Could you check a few things on this model? Use its own coordinates, in mm. A direction names the side the tool comes from. Give positions to 0.01 mm unless a question says otherwise; leave off trailing zeros. Order: outer loops, then holes, each group sorted by start corner. A loop starts at its lowest first (then second) coordinate and runs counter-clockwise, first axis right, second up. Notation, with made-up numbers: (44.25, 60) - (71.25, 60) arc R32 cw to (71.25, 91) - close; hole circle Ø4 at (39, 27). An arc over 180 degrees is marked (long way). One line per question, with ' | ' between items. Start each with the question number.
1. Imagine slicing it at B-B (x = 9). Please give me the cut outline in (y, z), and give its area (3 significant figures).
2. Which directions (+Z, -Z, +X, -X, +Y, -Y) give clear straight access to the entire face, cutting with the end or side of a thin tool? Please do faces 5 (the flat face through (50, -1, 12)), 6 (the flat face through (-1, -40, 24)).
3. For P1, Ø4, axis at x = 21.5, y = -9.5, coming from the +Z side; P2, Ø10, axis at x = -36.5, y = -38.5, coming from the -Z side, each with a flat end and sliding along its axis, tell me the tip position at first contact or that it passes through.
4. I need wall thicknesses on probe 1 along X at (y, z) = (18, 4); probe 2 along Z at (x, y) = (-21, 46.5). Which ranges of each line are inside material? Lowest first, please. Write a range as from..to.
5. Imagine slicing it at D-D (z = 20.25). Please give me the cut outline in (x, y).
6. Imagine slicing it at C-C (y = -26). Please give me the cut outline in (x, z), and give its area (4 significant figures).
7. If we mould it in two halves opening along Z, with no side actions, what happens to faces 1 (the flat face through (-1, 50, 12)), 2 (the flat face through (0, 49, 25)), 3 (the flat face through (-1, -47.5, 9)), 4 (the cylindrical face through (0.665, -45.361, 20.245))? For each: released by +Z, released by -Z, zero draft, split by the parting line, or undercut.
8. Imagine slicing it at A-A (z = 8). Please give me the cut outline in (x, y).
```python
from build123d import *

# Parameters (mm, degrees)
F0_W     = 100
F0_H     = 100
F1_DEPTH = 25
F2_R     = 10
F3_T     = -2.5


# Not quite as in the source:
# - a shell that OpenCascade refuses in one call is made with other operations: the cavity is built on its own and cut out


with BuildPart() as f1:
    # F0 (on Top) → F1 (new body)
    with BuildSketch(Plane.XY):
        Rectangle(F0_W, F0_H)
    extrude(amount=F1_DEPTH)

    # F2
    f2_edges = [f1.edges().sort_by_distance(p)[0] for p in [
        (0, -50, 25),
    ]]
    fillet(f2_edges, radius=F2_R)

    # F3: a shell. OpenCascade refuses it in one call, so the cavity is built on its own and cut out:
    # the body offset inwards by the wall thickness, plus a prism from it out through each open face.
    f3_core = offset(f1.part, amount=F3_T, mode=Mode.PRIVATE)
    f3_exits = [f3_core.faces().sort_by_distance(p)[0] for p in [
        (0, 3.75, 22.5),
    ]]
    add(f3_core, mode=Mode.SUBTRACT)
    extrude(f3_exits, amount=-F3_T, mode=Mode.SUBTRACT)


solid = f1.part
```
Results found:
1) outline: (-50, 0) - (50, 0) - (50, 25) - (47.5, 25) - (47.5, 2.5) - (-47.5, 2.5) - (-47.5, 15) arc R7.5 cw to (-40, 22.5) - (-40, 25) arc R10 ccw to (-50, 15) - close | area: 372 mm2
2) face 5: +Z, -Z, +X, +Y, -Y | face 6: +Z
3) P1: stops at z = 2.5 | P2: stops at z = 0
4) probe 1: x = -50..-47.5, 47.5..50 | probe 2: z = 0..2.5
5) outline: (-50, -48.51) - (50, -48.51) - (50, 50) - (-50, 50) - close; hole (-47.5, -45.36) - (47.5, -45.36) - (47.5, 47.5) - (-47.5, 47.5) - close
6) outline: (-50, 0) - (50, 0) - (50, 25) - (47.5, 25) - (47.5, 2.5) - (-47.5, 2.5) - (-47.5, 25) - (-50, 25) - close | area: 362.5 mm2
7) face 1: zero draft | face 2: released by +Z | face 3: undercut | face 4: undercut
8) outline: (-50, -50) - (50, -50) - (50, 50) - (-50, 50) - close; hole (-47.5, -47.5) - (47.5, -47.5) - (47.5, 47.5) - (-47.5, 47.5) - close
